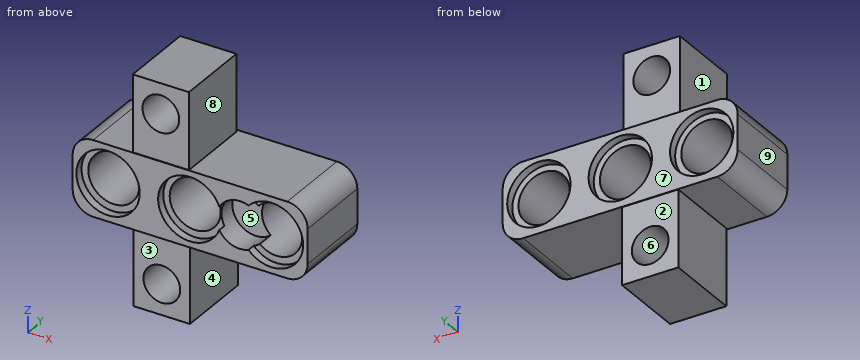
from build123d import *

# Parameters (mm, degrees)
SKETCH3_W           = 23
SKETCH3_H           = 7.38
BOSS_EXTRUDE1_DEPTH = 7.76
SKETCH4_R           = 3.1
CUT_EXTRUDE2_DEPTH  = 0.8
SKETCH7_R           = 3.1
CUT_EXTRUDE3_DEPTH  = 0.8
SKETCH6_R           = 2.5
CUT_EXTRUDE4_DEPTH  = 7.96
FILLET3_R           = 2
FILLET4_R           = 2
FILLET5_R           = 2
FILLET6_R           = 2
SKETCH8_W           = 5.5
SKETCH8_H           = 7.500541727
BOSS_EXTRUDE2_DEPTH = 7.5
SKETCH12_W          = 5.5
SKETCH12_H          = 7.41549866
BOSS_EXTRUDE4_DEPTH = 7.5
SKETCH9_R           = 1.8
CUT_EXTRUDE5_DEPTH  = 20.6
SKETCH13_R          = 1.8
CUT_EXTRUDE6_DEPTH  = 20.6
SKETCH14_R          = 2.3
CUT_EXTRUDE7_DEPTH  = 2.5


with BuildPart() as part:
    # Sketch3 → Boss-Extrude1 (new body)
    with BuildSketch(Plane(origin=(0, 0, 0), x_dir=(1, 0, 0), z_dir=(0, 1, 0))):
        with Locations((-11.5, 3.69)):
            Rectangle(SKETCH3_W, SKETCH3_H)
    extrude(amount=BOSS_EXTRUDE1_DEPTH)

    # Sketch4 → Cut-Extrude2 (cut)
    with BuildSketch(Plane(origin=(0, 0, 0), x_dir=(-1, 0, 0), z_dir=(0, -1, 0))):
        with Locations((19.538269405, 3.69)):
            Circle(SKETCH4_R)
        with Locations((11.538269405, 3.69)):
            Circle(SKETCH4_R)
        with Locations((3.538269405, 3.69)):
            Circle(SKETCH4_R)
    extrude(amount=-CUT_EXTRUDE2_DEPTH, mode=Mode.SUBTRACT)

    # Sketch7 → Cut-Extrude3 (cut)
    with BuildSketch(Plane(origin=(0, 7.76, 0), x_dir=(1, 0, 0), z_dir=(0, 1, 0))):
        with Locations((-19.478269405, 3.591470107)):
            Circle(SKETCH7_R)
        with Locations((-11.508269405, 3.591470107)):
            Circle(SKETCH7_R)
        with Locations((-3.538269405, 3.591470107)):
            Circle(SKETCH7_R)
    extrude(amount=-CUT_EXTRUDE3_DEPTH, mode=Mode.SUBTRACT)

    # Sketch6 → Cut-Extrude4 (cut, through all)
    with BuildSketch(Plane(origin=(0, 0.8, 0), x_dir=(-1, 0, 0), z_dir=(0, -1, 0))):
        with Locations((3.538269405, 3.591470107)):
            Circle(SKETCH6_R)
        with Locations((11.508269405, 3.591470107)):
            Circle(SKETCH6_R)
        with Locations((19.478269405, 3.591470107)):
            Circle(SKETCH6_R)
    extrude(amount=-CUT_EXTRUDE4_DEPTH, mode=Mode.SUBTRACT)

    # Fillet3
    fillet3_edges = [part.edges().sort_by_distance(p)[0] for p in [
        (0, 3.88, 0),
    ]]
    fillet(fillet3_edges, radius=FILLET3_R)

    # Fillet4
    fillet4_edges = [part.edges().sort_by_distance(p)[0] for p in [
        (-23, 3.88, 0),
    ]]
    fillet(fillet4_edges, radius=FILLET4_R)

    # Fillet5
    fillet5_edges = [part.edges().sort_by_distance(p)[0] for p in [
        (-23, 3.88, -7.38),
    ]]
    fillet(fillet5_edges, radius=FILLET5_R)

    # Fillet6
    fillet6_edges = [part.edges().sort_by_distance(p)[0] for p in [
        (0, 3.88, -7.38),
    ]]
    fillet(fillet6_edges, radius=FILLET6_R)

    # Sketch8 → Boss-Extrude2 (add)
    with BuildSketch(Plane(origin=(0, 0, -7.38), x_dir=(-1, 0, 0), z_dir=(0, 0, -1))):
        with Locations((14.4, 3.949980596)):
            Rectangle(SKETCH8_W, SKETCH8_H)
    extrude(amount=BOSS_EXTRUDE2_DEPTH)

    # Sketch12 → Boss-Extrude4 (add)
    with BuildSketch(Plane.XY):
        with Locations((-14.4, 3.755058696)):
            Rectangle(SKETCH12_W, SKETCH12_H)
    extrude(amount=BOSS_EXTRUDE4_DEPTH)

    # Sketch9 → Cut-Extrude5 (cut)
    with BuildSketch(Plane(origin=(0, 7.700251459, 0), x_dir=(1, 0, 0), z_dir=(0, 1, 0))):
        with Locations((-14.4, 11.902505055)):
            Circle(SKETCH9_R)
    extrude(amount=-CUT_EXTRUDE5_DEPTH, mode=Mode.SUBTRACT)

    # Sketch13 → Cut-Extrude6 (cut)
    with BuildSketch(Plane(origin=(0, 7.462808026, 0), x_dir=(1, 0, 0), z_dir=(0, 1, 0))):
        with Locations((-14.4, -4.550661236)):
            Circle(SKETCH13_R)
    extrude(amount=-CUT_EXTRUDE6_DEPTH, mode=Mode.SUBTRACT)

    # Sketch14 → Cut-Extrude7 (cut)
    with BuildSketch(Plane(origin=(0, 0, 0), x_dir=(-1, 0, 0), z_dir=(0, -1, 0))):
        with Locations((6.638269405, 3.69)):
            Circle(SKETCH14_R)
    extrude(amount=-CUT_EXTRUDE7_DEPTH, mode=Mode.SUBTRACT)


solid = part.part
The listing builds one solid part. Answer for the finished solid, in the listing's coordinates (mm). Face numbers are marked on the shaded views. A direction names the side the tool comes from. Coordinates: 2 decimals unless noted, no trailing zeros. Write each loop counter-clockwise with the first axis right and the second up, starting at its lowest first coordinate (ties: lowest second). Pieces come first, ordered by that corner, then holes. Notation, with made-up numbers: (7.25, 37) -> (42.25, 37) arc R15 cw to (42.25, 59) -> close; hole circle Ø6 at (-26, 58.25). An arc over 180 degrees is marked (long way). One line per question, with ' | ' between items.
1. Section C-C (y = 5.5) is taken. Determine the outline of the cut face in (x, z).
Verdict:
outline: (-23, -5.38) arc R2 ccw to (-21, -7.38) -> (-17.15, -7.38) -> (-17.15, -14.88) -> (-11.65, -14.88) -> (-11.65, -7.38) -> (-2, -7.38) arc R2 ccw to (0, -5.38) -> (0, -2) arc R2 ccw to (-2, 0) -> (-11.65, 0) -> (-11.65, 7.5) -> (-17.15, 7.5) -> (-17.15, 0) -> (-21, 0) arc R2 ccw to (-23, -2) -> close; hole circle Ø5 at (-19.48, -3.59); hole circle Ø3.6 at (-14.4, -11.9); hole circle Ø3.6 at (-14.4, 4.55); hole circle Ø5 at (-11.51, -3.59); hole circle Ø5 at (-3.54, -3.59)
2. Which of the six approach directions +Z, -Z, +X, -X, +Y, -Y give full straight-line access (tool end or side, diameter ignored) to the marked faces 1, 2, 3, 4 and 5?
Verdict:
face 1: +Z, -X, +Y, -Y | face 2: -Z, +X, -X, +Y | face 3: -Z, +X, -X, -Y | face 4: -Z, +X, +Y, -Y | face 5: -Y
3. Section B-B (y = 0.5) is taken. Determine the outline of the cut face in (x, z).
Verdict:
outline: (-23, -5.38) arc R2 ccw to (-21, -7.38) -> (-17.15, -7.38) -> (-17.15, -14.88) -> (-11.65, -14.88) -> (-11.65, -7.38) -> (-2, -7.38) arc R2 ccw to (0, -5.38) -> (0, -2) arc R2 ccw to (-2, 0) -> (-11.65, 0) -> (-11.65, 7.5) -> (-17.15, 7.5) -> (-17.15, 0) -> (-21, 0) arc R2 ccw to (-23, -2) -> close; hole circle Ø6.2 at (-19.54, -3.69); hole circle Ø3.6 at (-14.4, -11.9); hole circle Ø3.6 at (-14.4, 4.55); hole (-8.65, -4.81) arc R2.3 ccw to (-5.79, -5.83) arc R3.1 ccw (long way) to (-5.79, -1.55) arc R2.3 ccw to (-8.65, -2.57) arc R3.1 ccw (long way) to start
4. For a pull along X with two mould halves and no side action, classify the marked faces 6, 7, 8 and 9 as released by +X, released by -X, zero draft, split by the parting line, or undercut.
Verdict:
face 6: undercut | face 7: zero draft | face 8: released by +X | face 9: released by -X
5. Section D-D (y = 1.75) is taken. Determine the outline of the cut face in (x, z), and give its area (3 significant figures).
Verdict:
outline: (-23, -5.38) arc R2 ccw to (-21, -7.38) -> (-17.15, -7.38) -> (-17.15, -14.88) -> (-11.65, -14.88) -> (-11.65, -7.38) -> (-2, -7.38) arc R2 ccw to (0, -5.38) -> (0, -2) arc R2 ccw to (-2, 0) -> (-11.65, 0) -> (-11.65, 7.5) -> (-17.15, 7.5) -> (-17.15, 0) -> (-21, 0) arc R2 ccw to (-23, -2) -> close; hole circle Ø5 at (-19.48, -3.59); hole circle Ø3.6 at (-14.4, -11.9); hole circle Ø3.6 at (-14.4, 4.55); hole circle Ø5 at (-11.51, -3.59); hole (-5.3, -1.82) arc R2.3 ccw (long way) to (-5.18, -5.47) arc R2.5 ccw (long way) to start | area: 157 mm^2
6. Section A-A (x = -10.25) is taken. Determine the outline of the cut face in (y, z).
Verdict:
outline: (0, -7.38) -> (7.76, -7.38) -> (7.76, -6.42) -> (6.96, -6.42) -> (6.96, -5.75) -> (0.8, -5.75) -> (0.8, -6.51) -> (0, -6.51) -> close; (0, -0.87) -> (0.8, -0.87) -> (0.8, -1.43) -> (6.96, -1.43) -> (6.96, -0.76) -> (7.76, -0.76) -> (7.76, 0) -> (0, 0) -> close
7. Straight lines are drawn through the part: line 1 (X direction, y = 3, z = -3.75); line 2 (Z direction, x = -3.5, y = 1.5); line 3 (X direction, y = 6.5, z = -12). For each, find the intervals that lie inside material, in ascending order.
Verdict:
line 1: x = -23 to -21.97, -16.98 to -14, -9.01 to -6.03, -1.04 to 0 | line 2: z = -7.38 to -6.09, -1.09 to 0 | line 3: x = -17.15 to -16.2, -12.6 to -11.65
8. Given pin 1 Ø3 at (x, z) = (-3.54, -3.59) entering from +Y; pin 2 Ø1 at (x, y) = (-10, 7) entering from -Z; pin 3 Ø4.5 at (x, z) = (-13, -12) entering from -Y; pin 4 Ø1.6 at (x, z) = (-13.5, 4) entering from -Y, each flat-ended and moving along its own axis, determine where each tip first touches the part or whether it passes through.
Verdict:
pin 1: passes through | pin 2: stops at z = -7.38 | pin 3: stops at y = 0.2 | pin 4: stops at y = 0.05
